Geometry check sheet. Reference: the model listing, model coordinates, mm. A direction names the side the tool comes from. Give positions to 0.01 mm unless a question says otherwise; leave off trailing zeros. Order: outer loops, then holes, each group sorted by start corner. A loop starts at its lowest first (then second) coordinate and runs counter-clockwise, first axis right, second up.
Autodesk Inventor part; units mm, degrees
ref_plane "YZ Plane" through (0, 0, 0) normal (1, 0, 0) x (0, 1, 0)
ref_plane "XZ Plane" through (0, 0, 0) normal (0, 1, 0) x (-1, 0, 0)
ref_plane "XY Plane" through (0, 0, 0) normal (0, 0, 1) x (1, 0, 0)
sketch "Sketch1" plane through (0, 0, 0) normal (0, 0, 1) x (1, 0, 0)
  line L0 (-15.5, 18) -> (19.5, 18)
  line L1 (19.5, 18) -> (19.5, -18)
  line L2 (19.5, -18) -> (-15.5, -18)
  line L3 (-15.5, -18) -> (-15.5, 18)
  point P0 (0, 0)
  dimension "d0" = 35
  dimension "d1" = 36
  dimension "d2" = 18
  dimension "d3" = 15.5
extrude "Extrusion1" add sketch "Sketch1" along normal blind 8
sketch "Sketch2" plane through (0, 0, 8) normal (0, 0, 1) x (1, 0, 0)
  line L0 (-15.5, 18) -> (19.5, 18)
  line L1 (19.5, 18) -> (19.5, -18)
  line L2 (19.5, -18) -> (-15.5, -18)
  line L3 (-15.5, -18) -> (-15.5, 18)
  line L4 (-15.5, -18) -> (-15.5, 18)
  line L5 (19.5, 18) -> (19.5, -18)
  line L6 (-15.5, 18) -> (19.5, 18)
  line L7 (19.5, -18) -> (-15.5, -18)
  line L8 (19.5, -18) -> (19.5, 18)
  point P0 (0, 0)
  dimension "d70" = 0
  dimension "d165" = 0
extrude "Extrusion2" add sketch "Sketch2" along normal blind 22.5
sketch "Sketch3" plane through (-15.5, -18, 0) normal (0, -1, 0) x (1, 0, 0)
  line L0 (7.85, 30.5) -> (7.35, 30.5)
  line L1 (7.85, 30.5) -> (8.35, 30.5)
  line L2 (35, 0) -> (0, 0)
  arc A0 (7.35, 20.7234) -> (8.35, 20.7234) centre (7.85, 16) ccw
  line L3 (7.35, 30.5) -> (7.35, 20.7234)
  line L4 (8.35, 30.5) -> (8.35, 20.7234)
  line L5 (35, 0) -> (35, 30.5)
  line L6 (35, 30.5) -> (0, 30.5)
  line L7 (0, 0) -> (0, 30.5)
  point P0 (15.5, 0)
  dimension "d16" = 0.5
  dimension "d17" = 0.5
  dimension "d63" = 9.4996
  dimension "d65" = 16
  dimension "d105" = 1
  dimension "d188" = 7.85
  dimension "d189" = 0.5
emboss "Emboss1" sketch "Sketch3" operation cut depth 50 direction (0, 1, 0) contours L1 L4 A0 L3 L0
sketch "Sketch13" plane through (0, 0, 0) normal (0, 0, -1) x (-1, 0, 0)
  line L0 (-13, -5.3) -> (11, -5.3)
  line L1 (15.5, 18) -> (-19.5, 18)
  line L2 (-19.5, 18) -> (-19.5, -18)
  line L3 (-19.5, -18) -> (15.5, -18)
  line L4 (15.5, -18) -> (15.5, 18)
  line L5 (-19.5, 18) -> (-19.5, -18)
  line L6 (-19.5, -5.3) -> (15.5, -5.3)
  point P0 (0, 0)
  dimension "d190" = 12.7
extrude "Extrusion5" [suppressed]
sketch "Sketch14" plane through (-15.5, -5.3, 0) normal (0, 1, 0) x (1, 0, 0)
  line L0 (0, 32) -> (35, 32)
  line L1 (35, 0) -> (35, 32)
  point P0 (15.5, 0)
  point P1 (9.5, 30)
  point P2 (28, 30)
  point P3 (32.75, 16)
  dimension "d109" = 2
  dimension "d110" = 2
  dimension "d111" = 2.25
  dimension "d112" = 9.5
  dimension "d113" = 7
  dimension "d114" = 16
hole "Press fit for D2mm_L5mm Dowel - pin to protrude 2mm" [suppressed]
sketch "Sketch21" plane through (0, 0, 0) normal (0, 0, -1) x (-1, 0, 0)
  circle A0 centre (-3.75, 0.2) radius 3
  circle A1 centre (-3.75, 0.2) radius 3 construction
  point P0 (0, 0)
  dimension "d185" = 6
sketch "Sketch22" plane through (-15.5, -18, 30.5) normal (-1, 0, 0) x (0, 0, 1)
  line L0 (-30.5, 36) -> (0, 36)
  line L1 (-30.5, 0) -> (-30.5, 36)
  line L2 (-30.5, 0) -> (0, 0)
  line L3 (0, 0) -> (0, 36)
  point P0 (-30.5, 18)
  point P1 (-4, 30)
  point P2 (-4, 18)
  point P3 (-4, 6)
  dimension "d191" = 4
  dimension "d192" = 4
  dimension "d193" = 4
  dimension "d194" = 6
  dimension "d195" = 6
  dimension "d196" = 18
hole "CBore for M2.5 screw" [suppressed]
sketch "Sketch24" plane through (-7.65, -18, 16) normal (0, -1, 0) x (1, 0, 0)
  circle A0 centre (21.4, -42.5) radius 0.7835
  circle A1 centre (21.4, -22.5) radius 0.7835
  circle A2 centre (1.4, -42.5) radius 0.7835
  circle A3 centre (1.4, -22.5) radius 0.7835
  point P0 (7.65, -16)
hole "CBore for M2 screw" [suppressed]
sketch "Sketch25" plane through (-7.65, -18, 16) normal (0, -1, 0) x (1, 0, 0)
  line L0 (-0.5, 4.7234) -> (-0.5, 14.5)
  line L1 (-0.5, 14.5) -> (-7.85, 14.5)
  line L2 (-7.85, -16) -> (-7.85, 14.5)
  line L3 (27.15, -16) -> (27.15, 14.5)
  line L4 (27.15, 14.5) -> (0.5, 14.5)
  line L5 (0.5, 14.5) -> (0.5, 4.7234)
  arc A0 (-0.5, 4.7234) -> (0.5, 4.7234) centre (0, 0) ccw
  line L6 (27.15, -48) -> (-7.85, -48)
  circle A1 centre (1.4, -42.5) radius 2.2
  circle A2 centre (21.4, -42.5) radius 1.2
  line L7 (1.4, -42.5) -> (21.4, -42.5) construction
  line L8 (11.4, -42.5) -> (11.4, 14.5) construction
  line L9 (0.5, 14.5) -> (27.15, 14.5)
  line L10 (27.15, -16) -> (-7.85, -16)
  point P0 (7.65, -16)
  point P1 (11.4, -23)
  point P2 (11.4, -40)
hole "Threaded hole for M2 screw" [suppressed]
sketch "Sketch27" plane through (-15.5, 18, 0) normal (0, 1, 0) x (1, 0, 0)
  arc A0 (8.35, -20.7234) -> (7.35, -20.7234) centre (7.85, -16) ccw
  line L0 (7.35, -30.5) -> (7.35, -20.7234)
  arc A1 (8.35, -20.7234) -> (7.35, -20.7234) centre (7.85, -16) ccw
  line L1 (8.35, -20.7234) -> (8.35, -30.5)
  line L2 (8.35, -30.5) -> (35, -30.5)
  line L3 (35, 0) -> (35, -30.5)
  line L4 (0, 0) -> (35, 0)
  line L5 (0, 0) -> (0, -30.5)
  line L6 (0, -30.5) -> (7.35, -30.5)
  line L7 (7.85, -16) -> (7.85, -30.5)
  line L8 (7.85, -30.5) -> (0, -30.5)
  line L9 (0, -30.5) -> (0, 0)
  line L10 (0, 0) -> (7.85, 0)
  line L11 (7.85, 0) -> (7.85, -16)
  point P0 (15.5, 0)
extrude "Extrusion7" cut sketch "Sketch27" against normal through all contours L11 L7 L8 L0 A0 | A0 L0 L6 L5 L4 L11
sketch "Sketch23" plane through (-7.65, -18, 20.7234) normal (-1, 0, 0) x (0, 0, 1)
  line L0 (0, 0) -> (-9.4732, 0) construction
  line L1 (-9.4732, 36) -> (0, 36) construction
  line L2 (-4.7366, 0) -> (-4.7366, 36) construction
  point P0 (-20.7234, 18)
  point P1 (5.7766, 30)
  point P2 (5.7766, 18)
  point P3 (5.7766, 6)
  point P4 (-15.2498, 30)
  point P5 (-15.2498, 18)
  point P6 (-15.2498, 6)
  point P7 (5.7766, 30)
  point P8 (5.7766, 18)
  point P9 (5.7766, 6)
  dimension "d227" = 10.5132
  dimension "d228" = 10.5132
  dimension "d229" = 10.5132
  dimension "d230" = 10.5132
  dimension "d231" = 10.5132
  dimension "d232" = 10.5132
  dimension "d233" = 6
  dimension "d234" = 6
  dimension "d235" = 18
  dimension "d236" = 30
  dimension "d237" = 18
  dimension "d238" = 30
hole "Threaded hole for M2.5 screw" at (-7.65, 12, 26.5) at (-7.65, 0, 26.5) at (-7.65, -12, 26.5) at (-7.65, 12, 5.4736) at (-7.65, 0, 5.4736) at (-7.65, -12, 5.4736) direction (1, 0, 0) diameter 2.013 depth 10 tip angle 118
sketch "Sketch29" plane through (19.5, 18, 30.5) normal (0, 1, 0) x (1, 0, 0)
  arc A0 (-26.65, 9.7766) -> (-27.15, 19.2498) centre (-27.15, 14.5) ccw
  point P0 (-19.5, 30.5)
  point P1 (-23.5, 3)
  point P2 (-18.5, 3)
  point P3 (-23.5, 26)
  point P4 (-18.5, 26)
  dimension "d241" = 11.5
  dimension "d242" = 11.5
  dimension "d243" = 11.5
  dimension "d244" = 11.5
  dimension "d245" = 3.65
  dimension "d246" = 3.65
  dimension "d247" = 8.65
  dimension "d248" = 8.65
hole "Hole18" at (-4, 18, 27.5) at (1, 18, 27.5) at (-4, 18, 4.5) at (1, 18, 4.5) direction (0, -1, 0) diameter 1.567 depth 3 tip angle 118
sketch "Sketch31" plane through (0, 0, 0) normal (0, 0, -1) x (-1, 0, 0)
  line L0 (7.65, 18) -> (-19.5, 18)
  line L1 (7.65, -18) -> (7.65, 18)
  line L2 (-19.5, 18) -> (7.65, 18)
  line L3 (7.65, 18) -> (7.65, -18)
  line L4 (7.65, -18) -> (-19.5, -18)
  line L5 (-19.5, -18) -> (-19.5, 18)
  line L6 (-19.5, 18) -> (7.65, 18)
  line L7 (7.65, 18) -> (7.65, -18)
  line L8 (7.65, -18) -> (-19.5, -18)
  line L9 (-19.5, -18) -> (-19.5, 18)
  point P0 (0, 0)
extrude "Extrusion8" add sketch "Sketch31" along normal blind 9.9003
hole "Hole19" [suppressed]
sketch "Sketch30" plane through (0, 0, 30.5) normal (0, 0, 1) x (1, 0, 0)
  circle A0 centre (8.5, 0.2) radius 3
  line L0 (19.5, 18) -> (19.5, -18)
  line L1 (-7.15, 18) -> (19.5, 18)
  circle A1 centre (8.5, 9.1803) radius 1.1674
  circle A2 centre (8.5, -8.7803) radius 1.2033
  point P0 (0, 0)
  dimension "d263" = 6
  dimension "d264" = 11
  dimension "d265" = 17.8
  dimension "d273" = 8.9803
  dimension "d274" = 8.9803
hole "Hole20" at (8.5, 0.2, 30.5) direction (0, 0, -1) diameter 6.756 end through all counterbore diameter 9.652 counterbore depth 8
hole "Hole21" at (8.5, 9.1803, 30.5) direction (0, 0, -1) diameter 4.496 end through all counterbore diameter 7.938 counterbore depth 8
hole "Hole22" at (8.5, -8.7803, 30.5) direction (0, 0, -1) diameter 4.496 end through all counterbore diameter 7.938 counterbore depth 8
equation "\"d2\" = 0.5 * d1"
properties part number "zgalvo_to_newport_stage" material "ALUMINUM, 6061-T651"
Q1. Cross-section at C-C, the plane z = 25. Record the boundary of the cut face in (x, y), and give its area (3 significant figures).
Q2. Gauge pin test, flat ends, axial feed: P1, Ø1.8, axis at y = -12, z = 5.47, coming from the -X side; P2, Ø10.5, axis at x = 8.5, y = 9.18, coming from the +Z side; P3, Ø1.4, axis at x = -4, z = 27.5, coming from the +Y side; P4, Ø3, axis at y = 12, z = 26.5, coming from the -X side. Record the tip position at first contact, or that the pin passes through.
Q3. Access from +Z, -Z, +X, -X, +Y, -Y to the whole of each face (thin tool, end or side, straight path). Record for faces 1 (the face through (6, 18, 11)), 2 (the face through (-2.58, -11.017, 5.255)), 3 (the face through (-4.66, 16.48, 4.92)), 4 (the face through (6.981, 10.837, 6.073)), 5 (the face through (10.2, -10.5, 22.5)).
Q4. Cross-section at A-A, the plane z = 1.5. Record the boundary of the cut face in (x, y).
Q5. Release check for a two-part mould opening along Z. For faces 6 (the face through (2.85, 0.008, 26.325)), 7 (the face through (-7.15, 0, 24)), 8 (the face through (10, 7, 22.5)) record: pulls with the +Z half, pulls with the -Z half, needs draft (parallel to the pull), parting line crosses it, or undercut.
Q6. Cross-section at B-B, the plane y = -14.5. Record the boundary of the cut face in (x, z), and give its area (3 significant figures).
Q7. Thickness scan on L1, parallel to Y at x = 8.5, z = 6; L2, parallel to Z at x = 0.25, y = 12; L3, parallel to Y at x = 11.75, z = 24. Record the ranges inside material, lowest first.
Answers follow:
1. outline: (-7.15, -18) - (19.5, -18) - (19.5, 18) - (-7.15, 18) - close; hole circle Ø9.65 at (8.5, 0.2); hole circle Ø7.94 at (8.5, -8.78); hole circle Ø7.94 at (8.5, 9.18)
1. area: 787 mm2
2. P1: stops at x = 2.41
2. P2: stops at z = 30.5
2. P3: stops at y = 14.95
2. P4: stops at x = -7.15
3. face 1: +Z, -Z, +X, -X, +Y
3. face 2: -X
3. face 3: +Y
3. face 4: +Z, -Z
3. face 5: +Z
4. outline: (-7.65, -18) - (19.5, -18) - (19.5, 18) - (-7.65, 18) - close; hole circle Ø6.76 at (8.5, 0.2); hole circle Ø4.5 at (8.5, -8.78); hole circle Ø4.5 at (8.5, 9.18)
5. face 6: undercut
5. face 7: needs draft
5. face 8: pulls with the +Z half
6. outline: (-7.65, -9.9) - (19.5, -9.9) - (19.5, 30.5) - (-7.15, 30.5) - (-7.15, 20.72) arc R4.75 cw to (-7.65, 11.25) - close
6. area: 1,060 mm2
7. L1: y = -18 to -11.03, -6.53 to -3.18, 3.58 to 6.93, 11.43 to 18
7. L2: z = -9.9 to 4.47, 6.48 to 25.49, 27.51 to 30.5
7. L3: y = -18 to -11.06, -6.5 to -3.37, 3.77 to 6.9, 11.46 to 18
